Drawing for the job (mm, zero at the part's lowest x, y, z). A direction names the side the tool comes from. Round coordinates to 2 decimals unless told otherwise and drop trailing zeros. Write each loop counter-clockwise with the first axis right and the second up, starting at its lowest first coordinate (ties: lowest second). Pieces come first, ordered by that corner, then holes.
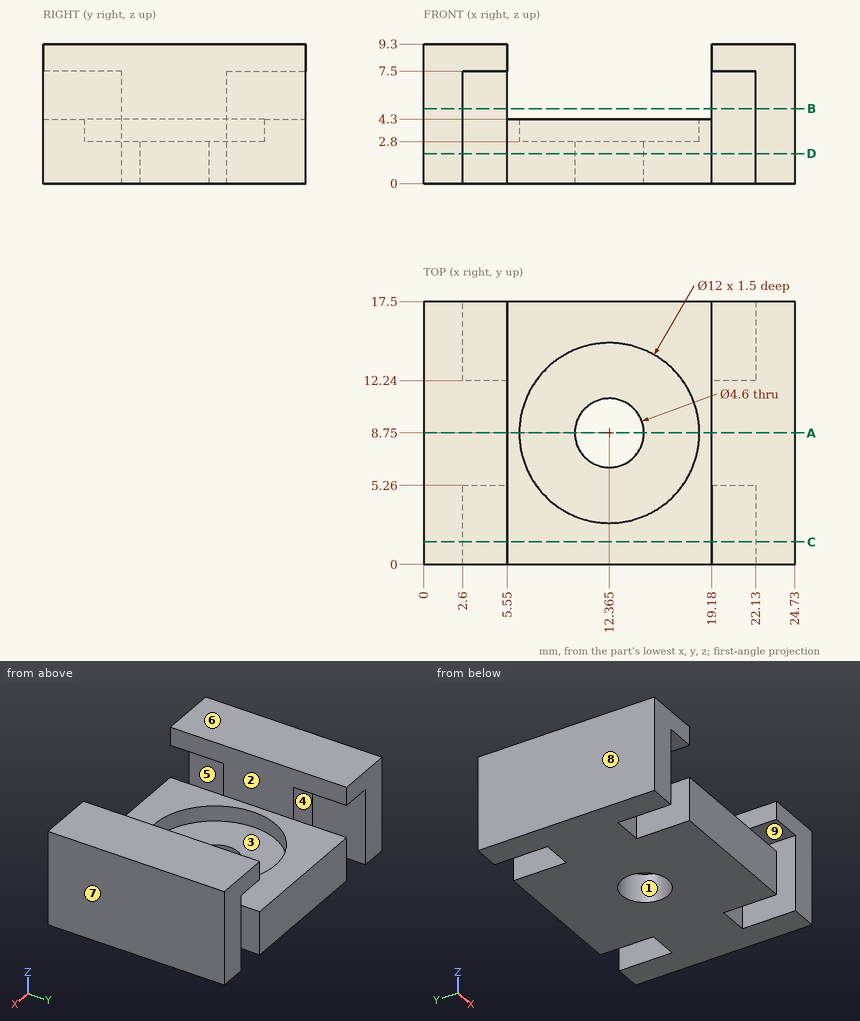
1) Cut at A-A on y = 8.75. List the corners of the cut face in (x, z) (3 decimals), and give its area (3 significant figures).
2) Flat gauge pins, fed straight in: pin 1 Ø1.5 at (x, z) = (20, 3) entering from +Y; pin 2 Ø2 at (x, y) = (4, 14.5) entering from -Z; pin 3 Ø3.5 at (x, y) = (13, 10) entering from +Z. Where does each tip first touch, or does it go through?
3) Wall check: probe 1 along X at (y, z) = (15.25, 4.25); probe 2 along X at (y, z) = (7, 4.5); probe 3 along X at (y, z) = (16.5, 4.75). Give the ranges that are in metal, low to high.
4) Pull direction X, two halves, no side cores. Call the marked faces 6, 7, 8 and 9: released by +X, released by -X, zero draft, split by the parting line, or undercut.
5) Which spindle directions (+Z, -Z, +X, -X, +Y, -Y) get a long thin tool onto all of the face, cutting with end or side? Do the marked faces 1, 2, 3, 4 and 5. Say none if no direction does.
6) Cut at B-B on z = 5. List the corners of the cut face in (x, y).
7) Cut at D-D on z = 2. List the corners of the cut face in (x, y) (3 decimals).
8) Cut at C-C on y = 1.5. List the corners of the cut face in (x, z), and give its area (3 significant figures).
Result sheet:
1. outline: (0, 0) - (10.065, 0) - (10.065, 2.8) - (6.365, 2.8) - (6.365, 4.3) - (5.55, 4.3) - (5.55, 9.3) - (0, 9.3) - close; (14.665, 0) - (24.73, 0) - (24.73, 9.3) - (19.18, 9.3) - (19.18, 4.3) - (18.365, 4.3) - (18.365, 2.8) - (14.665, 2.8) - close
1. area: 131 mm2
2. pin 1: stops at y = 12.24
2. pin 2: stops at z = 7.5
2. pin 3: stops at z = 2.8
3. probe 1: x = 0 to 2.6, 5.55 to 19.18, 22.13 to 24.73
3. probe 2: x = 0 to 5.55, 19.18 to 24.73
3. probe 3: x = 0 to 2.6, 22.13 to 24.73
4. face 6: zero draft
4. face 7: released by +X
4. face 8: released by -X
4. face 9: undercut
5. face 1: +Z, -Z
5. face 2: +Z, +Y, -Y
5. face 3: +Z
5. face 4: -Z, +Y
5. face 5: -Z, -Y
6. outline: (0, 0) - (2.6, 0) - (2.6, 5.26) - (5.55, 5.26) - (5.55, 12.24) - (2.6, 12.24) - (2.6, 17.5) - (0, 17.5) - close; (19.18, 5.26) - (22.13, 5.26) - (22.13, 0) - (24.73, 0) - (24.73, 17.5) - (22.13, 17.5) - (22.13, 12.24) - (19.18, 12.24) - close
7. outline: (0, 0) - (2.6, 0) - (2.6, 5.26) - (5.55, 5.26) - (5.55, 0) - (19.18, 0) - (19.18, 5.26) - (22.13, 5.26) - (22.13, 0) - (24.73, 0) - (24.73, 17.5) - (22.13, 17.5) - (22.13, 12.24) - (19.18, 12.24) - (19.18, 17.5) - (5.55, 17.5) - (5.55, 12.24) - (2.6, 12.24) - (2.6, 17.5) - (0, 17.5) - close; hole circle Ø4.6 at (12.365, 8.75)
8. outline: (0, 0) - (2.6, 0) - (2.6, 7.5) - (5.55, 7.5) - (5.55, 9.3) - (0, 9.3) - close; (5.55, 0) - (19.18, 0) - (19.18, 4.3) - (5.55, 4.3) - close; (19.18, 7.5) - (22.13, 7.5) - (22.13, 0) - (24.73, 0) - (24.73, 9.3) - (19.18, 9.3) - close
8. area: 118 mm2
